```python
from build123d import *

# Parameters (mm, degrees)
F0_R     = 58.4672149413
F1_DEPTH = 67.945
F2_R     = 12.7
F3_R     = 45.7672149413
F3_R_2   = 18.3189453451
F4_DEPTH = 25.4
F5_R     = 12.7


with BuildPart() as f1:
    # F0 (on Front) → F1 (new body)
    with BuildSketch(Plane.XZ):
        Circle(F0_R)
    extrude(amount=F1_DEPTH)

    # F2
    f2_edges = [f1.edges().sort_by_distance(p)[0] for p in [
        (-58.467215, -67.945, 0),
    ]]
    fillet(f2_edges, radius=F2_R)

    # F3 (on face) → F4 (cut)
    with BuildSketch(Plane.XZ.offset(67.945)):
        Circle(F3_R)
        Circle(F3_R_2, mode=Mode.SUBTRACT)
        Circle(F3_R_2)
    extrude(amount=-F4_DEPTH, mode=Mode.SUBTRACT)

    # F5
    f5_edges = [f1.edges().sort_by_distance(p)[0] for p in [
        (-45.767215, -42.545, 0),
    ]]
    fillet(f5_edges, radius=F5_R)


solid = f1.part
```
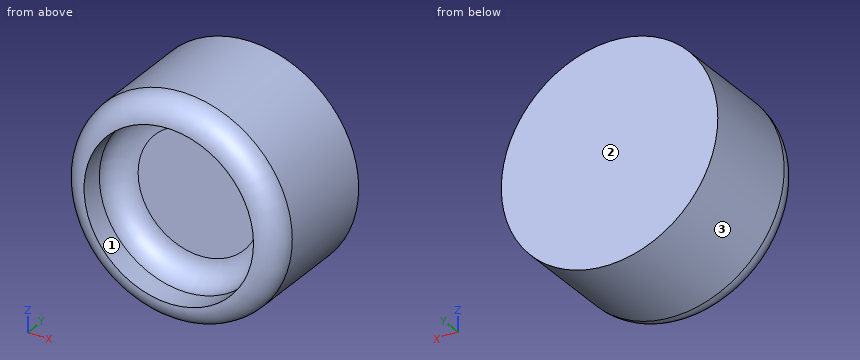
Could you check a few things on this model? Use its own coordinates, in mm. Face numbers are marked on the shaded views. Round coordinates to 2 decimals unless told otherwise and drop trailing zeros. Loops run counter-clockwise (first coordinate to the right, second up) from the corner with the lowest first, then second, coordinate; pieces in that order, holes last. Notation, with made-up numbers: (-8.5, 5) - (38.5, 5) arc R11 ccw to (38.5, 17) - close; hole circle Ø4 at (-15.75, 64). An arc over 180 degrees is marked (long way). Answer as CSV lines item,"result".
1. I want a section at B-B on z = 0. List the corners of the cut face in (x, y) for me (3 decimals), then the cut area to 3 significant figures.
Filled in:
outline,"(-58.467, -55.245) arc R12.7 ccw to (-45.767, -67.945) - (-45.767, -55.245) arc R12.7 cw to (-33.067, -42.545) - (33.067, -42.545) arc R12.7 cw to (45.767, -55.245) - (45.767, -67.945) arc R12.7 ccw to (58.467, -55.245) - (58.467, 0) - (-58.467, 0) - close"
area,"5,620 mm^2"
2. For pin 1 Ø3 at (x, y) = (16, -54.5) entering from +Z; pin 2 Ø1 at (x, y) = (37, -42.5) entering from +Z; pin 3 Ø12 at (x, y) = (-40.5, -17.5) entering from +Z, each with a flat end and sliding along its axis, tell me the tip position at first contact or that it passes through.
Filled in:
pin 1,"stops at z = 56.64"
pin 2,"stops at z = 45.67"
pin 3,"stops at z = 47.2"
3. We'd pull the mould along X, two halves only. Please class the marked faces 1, 2 and 3: +X half, -X half, draft (parallel to the pull), parting line (faces both ways), or undercut.
Filled in:
face 1,"undercut"
face 2,"draft"
face 3,"parting line"
4. I want a section at A-A on x = 0. List the corners of the cut face in (y, z) for me (3 decimals), then the cut area to 3 significant figures.
Filled in:
outline,"(-67.945, -45.767) arc R12.7 ccw to (-55.245, -58.467) - (0, -58.467) - (0, 58.467) - (-55.245, 58.467) arc R12.7 ccw to (-67.945, 45.767) - (-55.245, 45.767) arc R12.7 cw to (-42.545, 33.067) - (-42.545, -33.067) arc R12.7 cw to (-55.245, -45.767) - close"
area,"5,620 mm^2"
5. I want a section at C-C on y = -8. List the corners of the cut face in (x, z) for me.
Filled in:
outline,"circle Ø116.93 at (0, 0)"
6. Please list where these lines run through material, in increasing order: line 1 along Y through (x, z) = (28, 4) (3 decimals); line 2 along Z through (x, y) = (0, -59.5); line 3 along Z through (x, y) = (0, -65). Write a range as [from, to].
Filled in:
line 1,"y = [-42.545, 0]"
line 2,"z = [-57.73, -45.77], [45.77, 57.73]"
line 3,"z = [-53.9, -45.77], [45.77, 53.9]"
